Part print with two shaded views. Sizes in mm from the minimum x, y, z corner. Give positions to 0.01 mm unless a question says otherwise; leave off trailing zeros. Write each loop counter-clockwise with the first axis right and the second up, starting at its lowest first coordinate (ties: lowest second). Pieces come first, ordered by that corner, then holes.
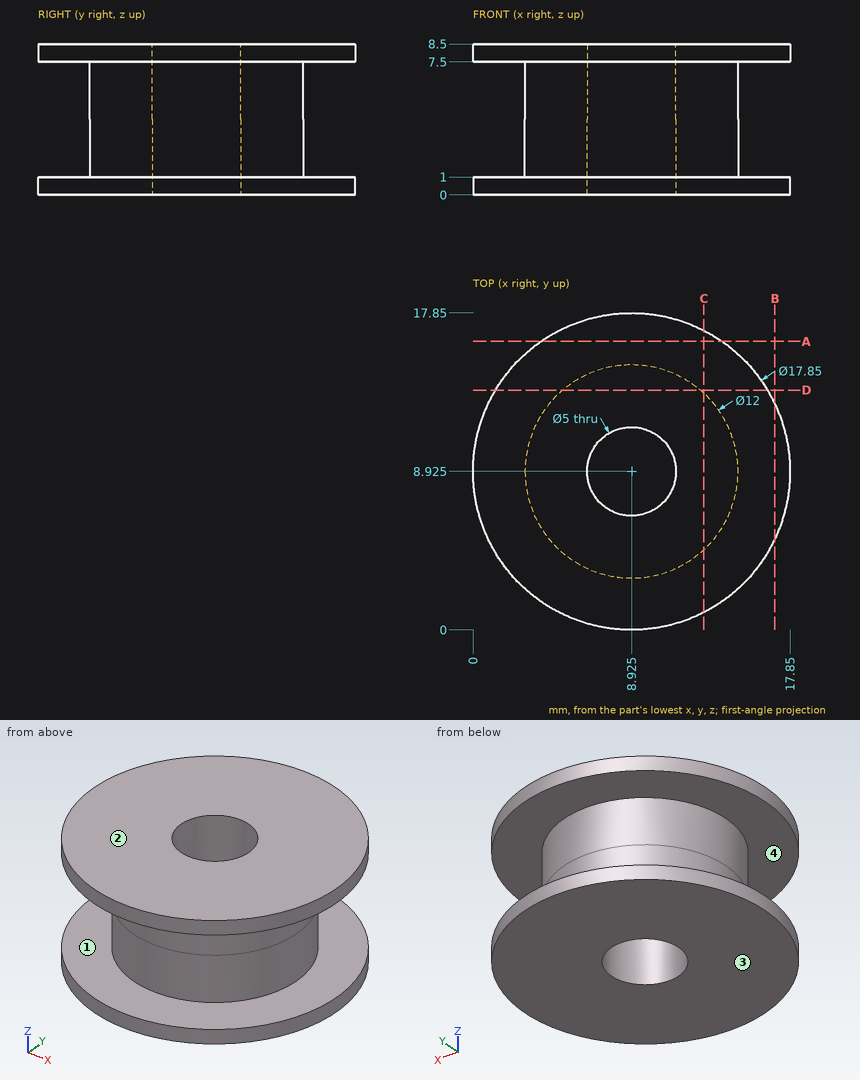
1) Saw through at D-D, the plane y = 13.5. Write the cut outline in (x, z).
Answers follow:
outline: (1.26, 0) - (16.59, 0) - (16.59, 1) - (12.81, 1) - (12.81, 7.5) - (16.59, 7.5) - (16.59, 8.5) - (1.26, 8.5) - (1.26, 7.5) - (5.04, 7.5) - (5.04, 1) - (1.26, 1) - close
2) Wall check: L1, parallel to Z at x = 3.25, y = 11.25; L2, parallel to Y at x = 10.5, z = 3.75; L3, parallel to Y at x = 6.75, z = 3. Give the ranges that are in metal, low to high.
Answers follow:
L1: z = 0 to 1, 7.5 to 8.5
L2: y = 3.14 to 6.98, 10.87 to 14.71
L3: y = 3.33 to 7.69, 10.16 to 14.52
3) Saw through at C-C, the plane x = 13. Write the cut outline in (y, z), then the cut area to 3 significant figures.
Answers follow:
outline: (0.98, 0) - (16.87, 0) - (16.87, 1) - (13.33, 1) - (13.33, 7.5) - (16.87, 7.5) - (16.87, 8.5) - (0.98, 8.5) - (0.98, 7.5) - (4.52, 7.5) - (4.52, 1) - (0.98, 1) - close
area: 89.0 mm2
4) Saw through at B-B, the plane x = 17. Write the cut outline in (y, z).
Answers follow:
outline: (5.12, 0) - (12.73, 0) - (12.73, 1) - (5.12, 1) - close; (5.12, 7.5) - (12.73, 7.5) - (12.73, 8.5) - (5.12, 8.5) - close
5) Saw through at A-A, the plane y = 16.25. Write the cut outline in (x, z).
Answers follow:
outline: (3.83, 0) - (14.02, 0) - (14.02, 1) - (3.83, 1) - close; (3.83, 7.5) - (14.02, 7.5) - (14.02, 8.5) - (3.83, 8.5) - close
6) Two-plate mould, pull along Z, no slides. Class the marked faces 1, 2, 3 and 4: +Z half, -Z half, draft (parallel to the pull), parting line (faces both ways), or undercut.
Answers follow:
face 1: undercut
face 2: +Z half
face 3: -Z half
face 4: undercut
7) Pin check, flat tips, straight feed: pin 1 Ø4 at (x, y) = (2.5, 9.5) entering from -Z; pin 2 Ø3 at (x, z) = (4.5, 3.5) entering from +Y. Stop position of each tip, or through.
Answers follow:
pin 1: stops at z = 0
pin 2: stops at y = 14.16
